```python
from build123d import *

# Parameters (mm, degrees)
CONG_1_R = 2.25


with BuildPart() as part:
    # Esquisse1 → Révolution1 (revolve)
    with BuildSketch(Plane.XY, mode=Mode.PRIVATE) as r_volution1_sk:
        Polygon((-27.993416317, 2.5), (-21.993416317, 2.5), (-21.993416317, 5.5), (-24.243416317, 5.5), (-24.243416317, 4), (-25.743416317, 4), (-25.743416317, 5.5), (-27.993416317, 5.5), align=None)
    revolve(r_volution1_sk.sketch.rotate(Axis((24.606805167, 0, 0), (-1, 0, 0)), 90), axis=Axis((24.606805167, 0, 0), (-1, 0, 0)))

    # Congé1
    cong_1_edges = [part.edges().sort_by_distance(p)[0] for p in [
        (-27.993416317, 0, 5.5),
        (-21.993416317, 0, 5.5),
    ]]
    fillet(cong_1_edges, radius=CONG_1_R - 0.0001)  # a hair under: the kernel refuses the full size


solid = part.part
```
Input: part model. Units: mm. Frame: model coordinates. A direction names the side the tool comes from. Coordinates: 2 decimals unless noted, no trailing zeros. Write each loop counter-clockwise with the first axis right and the second up, starting at its lowest first coordinate (ties: lowest second). Pieces come first, ordered by that corner, then holes.
1) Mould query, pull axis X, two halves, no side actions, for faces 1 (the cylindrical face through (-25.004, 3.905, 0.867)), 2 (the flat face through (-24.243, 2, 4)), 3 (the flat face through (-21.993, 2, 2)), 4 (the cylindrical face through (-25, -0.1, 2.5)). Classes: pulls with the +X half, pulls with the -X half, needs draft (parallel to the pull), parting line crosses it, or undercut.
2) Material intervals for line 1 along Y through (x, z) = (-24.7, 0); line 2 along Y through (x, z) = (-23.25, 0); line 3 along X through (y, z) = (-3, 4.25), sorted ascending.
3) Set-up query: faces 5 (the flat face through (-27.993, 2, -2)), 6 (the flat face through (-25.743, 2, -4)). Return all of +Z, -Z, +X, -X, +Y, -Y with unobstructed straight access to the full face (end or side cutting, diameter ignored); none if empty.
4) Section C-C on x = -24.4. Output: boundary loops of the cut face in (y, z).
5) Section D-D on x = -26.3. Output: boundary loops of the cut face in (y, z).
Check result:
1. face 1: undercut
1. face 2: undercut
1. face 3: pulls with the +X half
1. face 4: needs draft
2. line 1: y = -4 to -2.5, 2.5 to 4
2. line 2: y = -5.27 to -2.5, 2.5 to 5.27
2. line 3: x = -26.86 to -25.74, -24.24 to -23.12
3. face 5: +Z, -Z, -X, +Y, -Y
3. face 6: none
4. outline: circle Ø8 at (0, 0); hole circle Ø5 at (0, 0)
5. outline: circle Ø10.86 at (0, 0); hole circle Ø5 at (0, 0)
